```python
from build123d import *

# Parameters (mm, degrees)
F1_DEPTH = 6.35
F3_D     = 8.4328
F4_D     = 6.7564


with BuildPart() as f1:
    # F0 (on Front) → F1 (new body)
    with BuildSketch(Plane.XZ):
        with BuildLine():
            Line((-38.1, -12.7), (25.4, -12.7))
            ThreePointArc((25.4, -12.7), (34.380256, -8.980256), (38.1, 0))
            ThreePointArc((38.1, 0), (34.380256, 8.980256), (25.4, 12.7))
            Line((25.4, 12.7), (-38.1, 12.7))
            Line((-38.1, 12.7), (-38.1, -12.7))
        make_face()
    extrude(amount=F1_DEPTH)

    # F3 (through all)
    with Locations(Plane.XZ.offset(6.35)):
        with Locations((26.035, 0)):
            Hole(F3_D / 2)

    # F4 (through all)
    with Locations(Plane.XZ.offset(6.35)):
        with Locations((-25.4, 0), (-12.7, 0)):
            Hole(F4_D / 2)


solid = f1.part
```
CAD build for the part. Positions are in the model's coordinates, mm. Round coordinates to 2 decimals unless told otherwise and drop trailing zeros. Loops run counter-clockwise (first coordinate to the right, second up) from the corner with the lowest first, then second, coordinate; pieces in that order, holes last. Notation, with made-up numbers: M 80.25,-15 L 84.25,-15 A33 cw 84.25,22 Z; hole C -28,21 d8. An arc over 180 degrees is marked long. Return JSON: item names as keys, results as strings. Group by question number.
(1) Saw through at A-A, the plane z = -0.75. List the corners of the cut face in (x, y).
(2) Mould opens along X. For faces 1 (the flat face through (-7, -3, -12.7)), 2 (the cylindrical face through (-22.025, -3.131, 0.149)), 3 (the cylindrical face through (22.14, -3.13, -1.61)), 4 (the flat face through (-38.1, -3, 0)) say: +X half, -X half, draft (parallel to the pull), parting line (faces both ways), or undercut.
(3) Wall check: probe 1 along Z at (x, y) = (-25.4, -3.25); probe 2 along X at (y, z) = (-1.75, -2.75); probe 3 along X at (y, z) = (-1, -3.5). Give the ranges that are in metal, low to high. Write a range as [from, to].
(4) Saw through at D-D, the plane z = 11. List the corners of the cut face in (x, y), and give its area (3 significant figures).
(5) Saw through at B-B, the plane y = -3. List the corners of the cut face in (x, z) (3 decimals), and give its area (3 significant figures).
(6) Saw through at C-C, the plane x = -12.7. List the corners of the cut face in (y, z), and give its area (3 significant figures).
Answer list:
{
 "1": {"outline": "M -38.1,-6.35 L -28.69,-6.35 L -28.69,0 L -38.1,0 Z; M -22.11,-6.35 L -15.99,-6.35 L -15.99,0 L -22.11,0 Z; M -9.41,-6.35 L 21.89,-6.35 L 21.89,0 L -9.41,0 Z; M 30.18,-6.35 L 38.08,-6.35 L 38.08,0 L 30.18,0 Z"},
 "2": {"face 1": "draft", "face 2": "undercut", "face 3": "undercut", "face 4": "-X half"},
 "3": {"probe 1": "[-12.7, -3.38], [3.38, 12.7]", "probe 2": "[-38.1, -27.36], [-23.44, -14.66], [-10.74, 22.84], [29.23, 37.8]", "probe 3": "[-38.1, 23.68], [28.39, 37.61]"},
 "4": {"outline": "M -38.1,-6.35 L 31.75,-6.35 L 31.75,0 L -38.1,0 Z", "area": "444 mm2"},
 "5": {"outline": "M -38.1,-12.7 L 25.4,-12.7 A12.7 ccw 25.4,12.7 L -38.1,12.7 Z; hole C -25.4,0 d6.756; hole C -12.7,0 d6.756; hole C 26.035,0 d8.433", "area": "1,740 mm2"},
 "6": {"outline": "M -6.35,-12.7 L 0,-12.7 L 0,-3.38 L -6.35,-3.38 Z; M -6.35,3.38 L 0,3.38 L 0,12.7 L -6.35,12.7 Z", "area": "118 mm2"}
}
